Drawing for the job (mm, zero at the part's lowest x, y, z). Round coordinates to 2 decimals unless told otherwise and drop trailing zeros. Write each loop counter-clockwise with the first axis right and the second up, starting at its lowest first coordinate (ties: lowest second). Pieces come first, ordered by that corner, then holes.
Item 1: Band-saw the part on D-D, the plane z = 29.5. Write the cut outline in (x, y).
Item 2: Band-saw the part on B-B, the plane z = 39. Write the cut outline in (x, y).
Item 3: Band-saw the part on A-A, the plane y = 20. Write the cut outline in (x, z).
Item 4: Drop flat-ended pins along their axis: pin 1 Ø8 at (x, z) = (31.5, 9) entering from -Y; pin 2 Ø1 at (y, z) = (25, 10.5) entering from +X; pin 3 Ø6.5 at (x, z) = (20, 39) entering from -Y. Give the stop position or say it passes through.
Item 5: Mould opens along Y. For the marked faces 1, 2 and 3 say: +Y half, -Y half, draft (parallel to the pull), parting line (faces both ways), or undercut.
Item 6: Wall check: probe 1 along X at (y, z) = (19.5, 36); probe 2 along Y at (x, z) = (28, 33.5); probe 3 along X at (y, z) = (14.5, 24). Give the ranges that are in metal, low to high.
Item 7: Band-saw the part on C-C, the plane x = 20. Write the cut outline in (y, z).
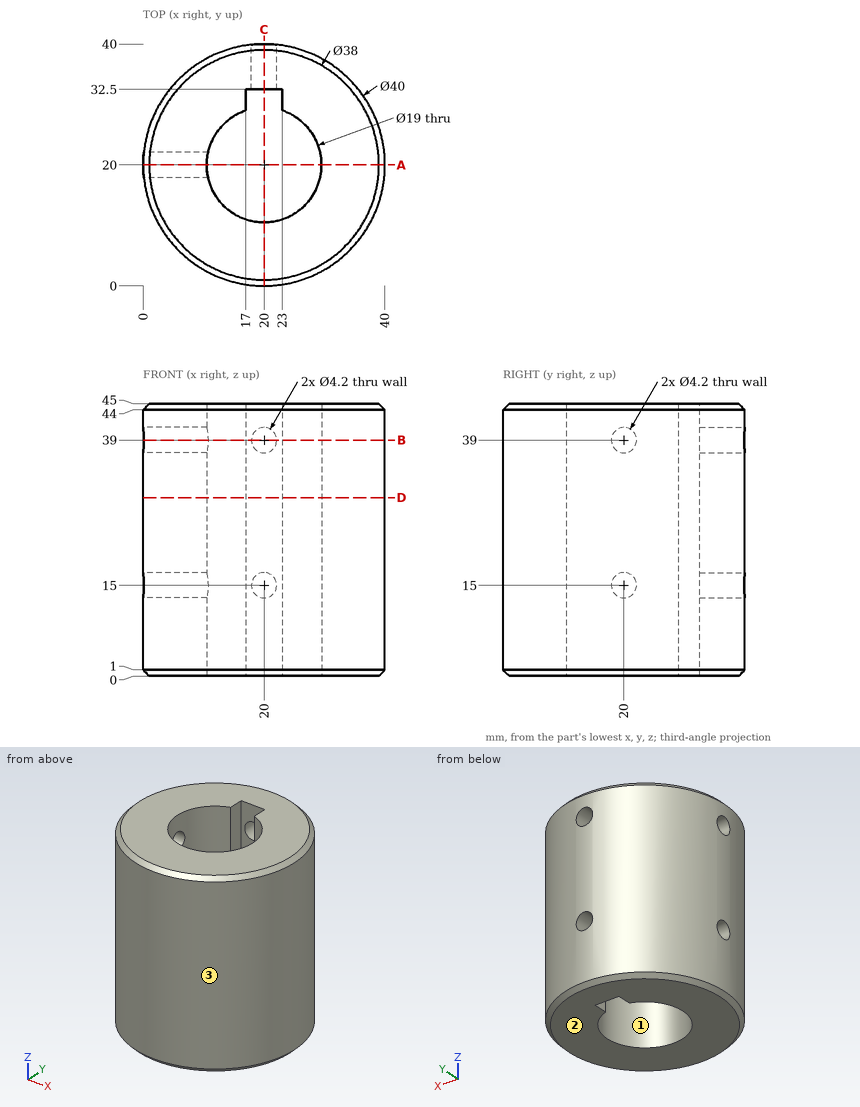
Results:
1. outline: circle Ø40 at (20, 20); hole (17, 29.01) arc R9.5 ccw (long way) to (23, 29.01) - (23, 32.5) - (17, 32.5) - close
2. outline: (0.11, 17.9) arc R20 ccw (long way) to (22.1, 39.89) - (22.1, 32.5) - (23, 32.5) - (23, 29.01) arc R9.5 cw (long way) to (10.74, 17.9) - close; (0.11, 22.1) - (10.74, 22.1) arc R9.5 cw to (17, 29.01) - (17, 32.5) - (17.9, 32.5) - (17.9, 39.89) arc R20 ccw to start
3. outline: (0, 1) - (1, 0) - (10.5, 0) - (10.5, 12.9) - (0, 12.9) - close; (0, 17.1) - (10.5, 17.1) - (10.5, 36.9) - (0, 36.9) - close; (0, 41.1) - (10.5, 41.1) - (10.5, 45) - (1, 45) - (0, 44) - close; (29.5, 0) - (39, 0) - (40, 1) - (40, 44) - (39, 45) - (29.5, 45) - close
4. pin 1: stops at y = 1.46
4. pin 2: stops at x = 39.49
4. pin 3: stops at y = 0
5. face 1: undercut
5. face 2: draft
5. face 3: parting line
6. probe 1: x = 0.01 to 10.51, 29.49 to 39.99
6. probe 2: y = 1.67 to 14.88, 25.12 to 38.33
6. probe 3: x = 0.77 to 12.25, 27.75 to 39.23
7. outline: (0, 1) - (1, 0) - (10.5, 0) - (10.5, 45) - (1, 45) - (0, 44) - close; (32.5, 0) - (39, 0) - (40, 1) - (40, 12.9) - (32.5, 12.9) - close; (32.5, 17.1) - (40, 17.1) - (40, 36.9) - (32.5, 36.9) - close; (32.5, 41.1) - (40, 41.1) - (40, 44) - (39, 45) - (32.5, 45) - close
